```python
from build123d import *

# Parameters (mm, degrees)
SKETCH_1_W          = 87.6
SKETCH_1_H          = 35.6
SKETCH_1_W_2        = 86
SKETCH_1_H_2        = 34
EXTRUDE_1_DEPTH     = 43
CHAMFER_1_SIZE      = 4
EXTRUDE_2_DEPTH     = 1
CUT_EXTRUDE_1_DEPTH = 65.585447277
FILLET_1_R          = 1.5
SKETCH_4_R          = 1.5
CUT_EXTRUDE_2_DEPTH = 64.908371909
SKETCH_5_W          = 12
SKETCH_5_H          = 44
EXTRUDE_3_DEPTH     = 6
SKETCH_6_W          = 2.5
SKETCH_6_H          = 3
CUT_EXTRUDE_3_DEPTH = 67.48969845
SKETCH_7_R          = 4
CUT_EXTRUDE_4_DEPTH = 2.2


with BuildPart() as part:
    # 草圖1 → 填料-伸長1 (new body)
    with BuildSketch(Plane.XY):
        Rectangle(SKETCH_1_W, SKETCH_1_H)
        Rectangle(SKETCH_1_W_2, SKETCH_1_H_2, mode=Mode.SUBTRACT)
    extrude(amount=EXTRUDE_1_DEPTH)

    # 導角1
    chamfer_1_edges = [part.edges().sort_by_distance(p)[0] for p in [
        (-43, 17, 21.5),
        (-43, -17, 21.5),
        (43, -17, 21.5),
        (43, 17, 21.5),
        (-43.8, 17.8, 21.5),
        (43.8, 17.8, 21.5),
        (43.8, -17.8, 21.5),
        (-43.8, -17.8, 21.5),
    ]]
    chamfer(chamfer_1_edges, length=CHAMFER_1_SIZE)

    # 草圖2 → 填料-伸長2 (add)
    with BuildSketch(Plane.XY.offset(43)):
        Polygon((-43.8, 13.8), (-39.8, 17.8), (39.8, 17.8), (43.8, 13.8), (43.8, -13.8), (39.8, -17.8), (-39.8, -17.8), (-43.8, -13.8), align=None)
    extrude(amount=EXTRUDE_2_DEPTH)

    # 草圖3 → 除料-伸長1 (cut, through all)
    with BuildSketch(Plane.XY.offset(44)):
        Polygon((15, -10), (40, -10), (40, 10), (-40, 10), (-40, -10), (-15, -10), (-15, -15), (15, -15), align=None)
    extrude(amount=-CUT_EXTRUDE_1_DEPTH, mode=Mode.SUBTRACT)

    # 圓角1
    fillet_1_edges = [part.edges().sort_by_distance(p)[0] for p in [
        (-40, -10, 43.5),
        (-40, 10, 43.5),
        (40, 10, 43.5),
        (40, -10, 43.5),
        (15, -10, 43.5),
        (15, -15, 43.5),
        (-15, -15, 43.5),
        (-15, -10, 43.5),
    ]]
    fillet(fillet_1_edges, radius=FILLET_1_R)

    # 草圖4 → 除料-伸長2 (cut, through all)
    with BuildSketch(Plane(origin=(0, 0, 43), x_dir=(-1, 0, 0), z_dir=(0, 0, -1))):
        with Locations((-38.75, 12.75)):
            Circle(SKETCH_4_R)
        with Locations(Location((38.75, 12.75, 0), (0, 0, 180))):
            Circle(SKETCH_4_R)
        with Locations((38.75, -12.75)):
            Circle(SKETCH_4_R)
        with Locations(Location((-38.75, -12.75, 0), (0, 0, 180))):
            Circle(SKETCH_4_R)
    extrude(amount=-CUT_EXTRUDE_2_DEPTH, mode=Mode.SUBTRACT)

    # 草圖5 → 填料-伸長3 (add)
    with BuildSketch(Plane.XZ.offset(17.8)):
        with Locations((0, 22)):
            Rectangle(SKETCH_5_W, SKETCH_5_H)
    extrude(amount=EXTRUDE_3_DEPTH)

    # 草圖6 → 除料-伸長3 (cut, through all)
    with BuildSketch(Plane.XY.offset(44)):
        with Locations((4.75, -19.3)):
            Rectangle(SKETCH_6_W, SKETCH_6_H)
        with Locations((-4.75, -19.3)):
            Rectangle(SKETCH_6_W, SKETCH_6_H)
    extrude(amount=-CUT_EXTRUDE_3_DEPTH, mode=Mode.SUBTRACT)

    # 草圖7 → 除料-伸長4 (cut)
    with BuildSketch(Plane.XZ.offset(23.8)):
        with Locations(Location((0, 6, 0), (0, 0, 270))):
            Circle(SKETCH_7_R)
        with Locations(Location((0, 21, 0), (0, 0, 270))):
            Circle(SKETCH_7_R)
        with Locations(Location((0, 36, 0), (0, 0, 270))):
            Circle(SKETCH_7_R)
    extrude(amount=-CUT_EXTRUDE_4_DEPTH, mode=Mode.SUBTRACT)


solid = part.part
```
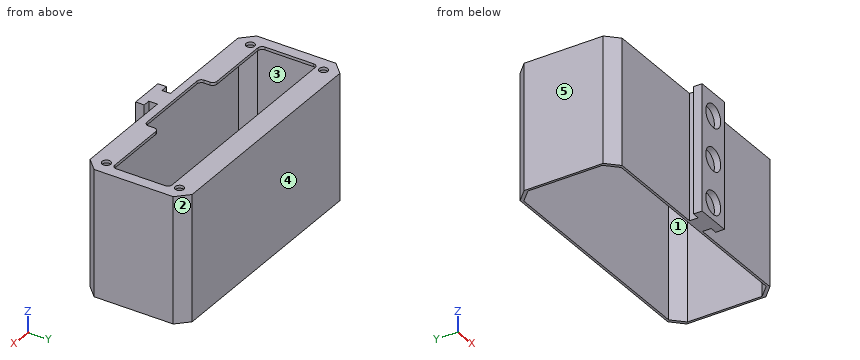
Check sheet for the modelled part. Datum: model origin and axes. Units: mm. Face numbers are marked on the shaded views. A direction names the side the tool comes from. Round coordinates to 2 decimals unless told otherwise and drop trailing zeros. Loops run counter-clockwise (first coordinate to the right, second up) from the corner with the lowest first, then second, coordinate; pieces in that order, holes last. Notation, with made-up numbers: (-26.75, 27.5) - (11.25, 27.5) arc R21 cw to (11.25, 51.5) - close; hole circle Ø11 at (44, 86.5). An arc over 180 degrees is marked (long way). Write item = value, one per line. Start each with the question number.
Q1. Release check for a two-part mould opening along Y. For the marked faces 3, 4 and 5 record: pulls with the +Y half, pulls with the -Y half, needs draft (parallel to the pull), parting line crosses it, or undercut.
Q2. Section check D-D (x = 31). Record the boundary of the cut face in (y, z), plus the area to 3 significant figures.
Q3. Thickness scan on L1, parallel to Y at x = -4.5, z = 39; L2, parallel to Y at x = 38.75, z = 43.75; L3, parallel to Y at x = -23, z = 8. Record the ranges inside material, lowest first.
Q4. Section check C-C (y = -6). Record the boundary of the cut face in (x, z).
Q5. Section check A-A (x = 0). Record the boundary of the cut face in (y, z), plus the area to 3 significant figures.
Q6. Depth check by flat-ended pin: P1, Ø3, axis at x = 7.5, y = -18.5, coming from the +Z side; P2, Ø4, axis at x = 32.5, y = 12.5, coming from the -Z side; P3, Ø3.5, axis at y = -19.5, z = 18, coming from the -X side; P4, Ø1.5, axis at y = -19.5, z = 15.5, coming from the +X side. Enter the tip coordinate at first touch or a pass-through.
Q7. Section check B-B (z = 36). Record the boundary of the cut face in (x, y), plus the area to 3 significant figures.
Q8. Access from +Z, -Z, +X, -X, +Y, -Y to the whole of each face (thin tool, end or side, straight path). Record for the marked faces 1 and 2.
Derived:
q1.face_3 = undercut
q1.face_4 = pulls with the +Y half
q1.face_5 = needs draft
q2.outline = (-17.8, 0) - (-17, 0) - (-17, 43) - (-10, 43) - (-10, 44) - (-17.8, 44) - close; (10, 43) - (17, 43) - (17, 0) - (17.8, 0) - (17.8, 44) - (10, 44) - close
q2.area = 84.4 mm^2
q3.L1 = -23.8 to -20.8, -17.8 to -17, 17 to 17.8
q3.L2 = -17.8 to -14.25, -11.25 to -9.98, 9.98 to 11.25, 14.25 to 17.8
q3.L3 = -17.8 to -17, 17 to 17.8
q4.outline = (-43.8, 0) - (-43, 0) - (-43, 43) - (-40, 43) - (-40, 44) - (-43.8, 44) - close; (40, 43) - (43, 43) - (43, 0) - (43.8, 0) - (43.8, 44) - (40, 44) - close
q5.outline = (-23.8, 0) - (-17, 0) - (-17, 43) - (-15, 43) - (-15, 44) - (-23.8, 44) - (-23.8, 40) - (-21.6, 40) - (-21.6, 32) - (-23.8, 32) - (-23.8, 25) - (-21.6, 25) - (-21.6, 17) - (-23.8, 17) - (-23.8, 10) - (-21.6, 10) - (-21.6, 2) - (-23.8, 2) - close; (10, 43) - (17, 43) - (17, 0) - (17.8, 0) - (17.8, 44) - (10, 44) - close
q5.area = 291 mm^2
q6.P1 = 44
q6.P2 = 43
q6.P3 = -39.85
q6.P4 = 3.5
q7.outline = (-43.8, -13.8) - (-39.8, -17.8) - (-3.5, -17.8) - (-3.5, -20.8) - (-6, -20.8) - (-6, -23.8) - (-4, -23.8) - (-4, -21.6) - (4, -21.6) - (4, -23.8) - (6, -23.8) - (6, -20.8) - (3.5, -20.8) - (3.5, -17.8) - (39.8, -17.8) - (43.8, -13.8) - (43.8, 13.8) - (39.8, 17.8) - (-39.8, 17.8) - (-43.8, 13.8) - close; hole (-43, -13) - (-39, -17) - (39, -17) - (43, -13) - (43, 13) - (39, 17) - (-39, 17) - (-43, 13) - close
q7.area = 234 mm^2
q8.face_1 = -Z
q8.face_2 = +Z, -Z, +X, +Y
